Design review of the part built by this model. Coordinates are the model's own, in mm. Coordinates: 2 decimals unless noted, no trailing zeros. Loops run counter-clockwise (first coordinate to the right, second up) from the corner with the lowest first, then second, coordinate; pieces in that order, holes last. Notation, with made-up numbers: (74, -1.5) -> (95, -1.5) arc R21 ccw to (95, 17.5) -> close; hole circle Ø6 at (9, -31.75). An arc over 180 degrees is marked (long way). Answer as a JSON object with one key per item and string values.
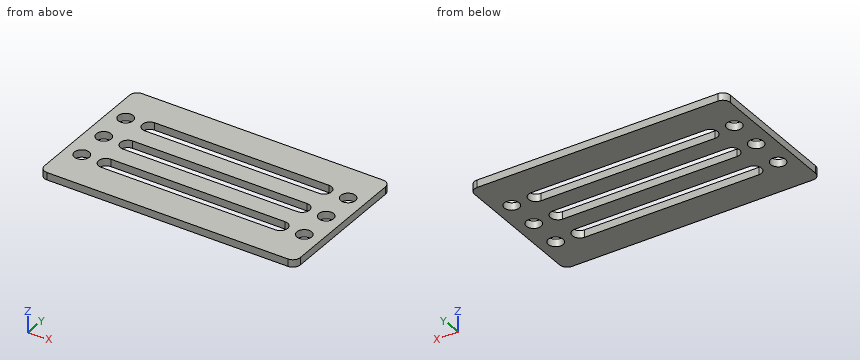
Autodesk Inventor part; units mm, degrees
ref_plane "YZ Plane" through (0, 0, 0) normal (1, 0, 0) x (0, 1, 0)
ref_plane "XZ Plane" through (0, 0, 0) normal (0, 1, 0) x (-1, 0, 0)
ref_plane "XY Plane" through (0, 0, 0) normal (0, 0, 1) x (1, 0, 0)
sketch "Эскиз1" plane through (0, 0, 0) normal (0, 0, 1) x (1, 0, 0)
  line L0 (-28.98, 25.9133) -> (40.02, 25.9133)
  line L1 (40.02, 25.9133) -> (40.02, -13.0867)
  line L2 (40.02, -13.0867) -> (-28.98, -13.0867)
  line L3 (-28.98, -13.0867) -> (-28.98, 25.9133)
  arc A0 (-17.98, 8.4133) -> (-17.98, 4.4133) centre (-17.98, 6.4133) ccw
  line L4 (-17.98, 8.4133) -> (5.52, 8.4133)
  line L5 (-17.98, 4.4133) -> (5.52, 4.4133)
  arc A1 (-17.98, 17.4133) -> (-17.98, 13.4133) centre (-17.98, 15.4133) ccw
  line L6 (-17.98, 17.4133) -> (5.52, 17.4133)
  line L7 (-17.98, 13.4133) -> (5.52, 13.4133)
  circle A2 centre (-24.48, 15.4133) radius 2
  circle A3 centre (-24.48, 6.4133) radius 2
  arc A4 (-17.98, -0.5867) -> (-17.98, -4.5867) centre (-17.98, -2.5867) ccw
  line L8 (-17.98, -4.5867) -> (5.52, -4.5867)
  line L9 (-17.98, -0.5867) -> (5.52, -0.5867)
  circle A5 centre (-24.48, -2.5867) radius 2
  arc A6 (29.02, 4.4133) -> (29.02, 8.4133) centre (29.02, 6.4133) ccw
  line L10 (29.02, 8.4133) -> (5.52, 8.4133)
  line L11 (29.02, 4.4133) -> (5.52, 4.4133)
  arc A7 (29.02, 13.4133) -> (29.02, 17.4133) centre (29.02, 15.4133) ccw
  line L12 (29.02, 17.4133) -> (5.52, 17.4133)
  line L13 (29.02, 13.4133) -> (5.52, 13.4133)
  circle A8 centre (35.52, 15.4133) radius 2
  circle A9 centre (35.52, 6.4133) radius 2
  circle A10 centre (35.52, -2.5867) radius 2
  line L14 (29.02, -4.5867) -> (5.52, -4.5867)
  arc A11 (29.02, -4.5867) -> (29.02, -0.5867) centre (29.02, -2.5867) ccw
  line L15 (29.02, -0.5867) -> (5.52, -0.5867)
  point P0 (0, 0)
  dimension "d0" = 69
  dimension "d1" = 39
  dimension "d3" = 4
  dimension "d8" = 4
  dimension "d9" = 4
extrude "Выдавливание1" add sketch "Эскиз1" along normal blind 2
fillet "Сопряжение1" radius 2 4 edges at (-28.98, 25.9133, 1) (40.02, 25.9133, 1) (40.02, -13.0867, 1) (-28.98, -13.0867, 1)
properties part number "радиатор"
1) Add section B-B, the plane z = 1.5. Count the separate pieces of the cut face and the enclosed holes in it, and give its area (3 significant figures).
Completed:
{"separate pieces": "1", "enclosed holes": "9", "area": "2,010 mm²"}
2) Wall thickness on probe 1 along Y at (x, z) = (14, 0.5); probe 2 along Y at (x, z) = (-23, 0.8); probe 3 along X at (y, z) = (17, 1.35): over which ranges is each line inside the solid? List them lowest first.
Completed:
{"probe 1": "-13.09 to -4.59, -0.59 to 4.41, 8.41 to 13.41, 17.41 to 25.91", "probe 2": "-13.09 to -3.93, -1.24 to 5.07, 7.76 to 14.07, 16.76 to 25.91", "probe 3": "-28.98 to -25.7, -23.26 to -19.2, 30.24 to 34.3, 36.74 to 40.02"}
3) Add section A-A, the plane x = 35.52. Give the boundary of the cut face in (y, z), and give its area (3 significant figures).
Completed:
{"outline": "(-13.09, 0) -> (-4.59, 0) -> (-4.59, 2) -> (-13.09, 2) -> close; (-0.59, 0) -> (4.41, 0) -> (4.41, 2) -> (-0.59, 2) -> close; (8.41, 0) -> (13.41, 0) -> (13.41, 2) -> (8.41, 2) -> close; (17.41, 0) -> (25.91, 0) -> (25.91, 2) -> (17.41, 2) -> close", "area": "54.0 mm²"}
